Input: part model. Units: mm. Frame: model coordinates. A direction names the side the tool comes from. Coordinates: 2 decimals unless noted, no trailing zeros. Write each loop counter-clockwise with the first axis right and the second up, starting at its lowest first coordinate (ties: lowest second). Pieces come first, ordered by that corner, then holes.
Autodesk Inventor part; units mm, degrees
ref_plane "YZ Plane" through (0, 0, 0) normal (1, 0, 0) x (0, 1, 0)
ref_plane "XZ Plane" through (0, 0, 0) normal (0, 1, 0) x (-1, 0, 0)
ref_plane "XY Plane" through (0, 0, 0) normal (0, 0, 1) x (1, 0, 0)
sketch "Sketch2" plane through (0, 0, 0) normal (0, 1, 0) x (-1, 0, 0)
  line L0 (-2.5, 6) -> (2.5, 6)
  line L1 (2.5, 6) -> (2.5, -6)
  line L2 (2.5, -6) -> (-2.5, -6)
  line L3 (-2.5, -6) -> (-2.5, 6)
  line L4 (-2.5, 6) -> (2.5, -6) construction
  line L5 (2.5, 6) -> (-2.5, -6) construction
  line L6 (2.5, 0) -> (-2.5, 0)
  circle A0 centre (0, 3) radius 0.8
  circle A1 centre (0, -3) radius 0.8
  line L7 (-5.5, -9) -> (5.5, -9)
  line L8 (5.5, -9) -> (5.5, 9)
  line L9 (5.5, 9) -> (-5.5, 9)
  line L10 (-5.5, 9) -> (-5.5, -9)
  line L11 (-5.5, -9) -> (5.5, 9) construction
  line L12 (5.5, -9) -> (-5.5, 9) construction
  point P0 (0, 0)
  dimension "d2" = 5
  dimension "d3" = 12
  dimension "d4" = 1.6
  dimension "d5" = 2.5
  dimension "d6" = 3
  dimension "d7" = 11
  dimension "d8" = 18
extrude "Extrusion2" add sketch "Sketch2" along normal blind 2 contours L0 L1 L6 L3 | L6 L1 L2 L3
extrude "Extrusion3" add sketch "Sketch2" along normal blind 5 contours L10 L9 L8 L7
fillet "Fillet1" radius 2 8 edges at (-5.5, 0, 0) (0, 0, -9) (5.5, 0, 0) (0, 0, 9) (-5.5, 2.5, -9) (-5.5, 2.5, 9) (5.5, 2.5, 9) (5.5, 2.5, -9)
sketch "Sketch4" plane through (-5.5, 0, -9) normal (-1, 0, 0) x (0, 0, 1)
  line L0 (0, 0) -> (18, 0) construction
  line L1 (18, 0) -> (18, 5) construction
  line L2 (0, 0) -> (18, 0) construction
  line L3 (18, 0) -> (18, 2) construction
  line L4 (18, 2) -> (0, 2) construction
  line L5 (0, 2) -> (0, 0) construction
  line L6 (9, 0) -> (9, 7)
  line L7 (0, 5) -> (18, 5) construction
  circle A0 centre (6, 4.5) radius 1
  circle A1 centre (12, 4.5) radius 1
  dimension "d13" = 2
  dimension "d15" = 2
  dimension "d16" = 6
  dimension "d17" = 2.5
properties part number "Part1_3DPrint"
Item 1: Section query B-B, the plane x = 0.5. Return loops of the section in (y, z), then the cut area to 3 significant figures.
Item 2: Pin query (flat end, axial travel): pin 1 Ø4 at (x, z) = (0, 0.5) entering from +Y; pin 2 Ø1.3 at (x, z) = (0, -3) entering from +Y. Return the tip coordinate at first contact, or that it passes through.
Item 3: Section query A-A, the plane y = 4. Return loops of the section in (x, z).
Item 4: Material intervals for line 1 (X direction, y = 4.7, z = 4.5); line 2 (Z direction, x = 0, y = 1.25); line 3 (Z direction, x = 0.25, y = 4.15), sorted ascending.
Item 5: Section query D-D, the plane z = -0.75. Return loops of the section in (x, y).
Item 6: Pull-direction query (Z, two-part tool) for faces 1 (the face through (5.5, 3, 0)), 2 (the face through (0.17, 0.99, 3.78)), 3 (the face through (0.05, 0.6, 8.43)), 4 (the face through (0, 2, 0)); classes: released by +Z, released by -Z, zero draft, split by the parting line, or undercut.
Item 7: Access query for faces 5 (the face through (0, 3, -6)), 6 (the face through (0, 0, 0)). Directions: +Z, -Z, +X, -X, +Y, -Y. A direction counts if a zero-diameter tool reaches every point of the face in a straight line with its end or side. Return the directions, or none.
Item 8: Section query C-C, the plane z = 3. Return loops of the section in (x, y).
The answers:
1. outline: (0, -7) arc R2 ccw to (2, -9) - (5, -9) - (5, -6) - (2, -6) - (2, -3.62) - (0, -3.62) - close; (0, -2.38) - (2, -2.38) - (2, 2.38) - (0, 2.38) - close; (0, 3.62) - (2, 3.62) - (2, 6) - (5, 6) - (5, 9) - (2, 9) arc R2 ccw to (0, 7) - close
1. area: 47.3 mm2
2. pin 1: stops at y = 2
2. pin 2: passes through
3. outline: (-5.5, -7) arc R2 ccw to (-3.5, -9) - (3.5, -9) arc R2 ccw to (5.5, -7) - (5.5, 7) arc R2 ccw to (3.5, 9) - (-3.5, 9) arc R2 ccw to (-5.5, 7) - close; hole (-2.5, -6) - (2.5, -6) - (2.5, 6) - (-2.5, 6) - close
4. line 1: x = -5.5 to -2.5, 2.5 to 5.5
4. line 2: z = -8.85 to -3.8, -2.2 to 2.2, 3.8 to 8.85
4. line 3: z = -9 to -6, 6 to 9
5. outline: (-5.5, 2) arc R2 ccw to (-3.5, 0) - (3.5, 0) arc R2 ccw to (5.5, 2) - (5.5, 5) - (2.5, 5) - (2.5, 2) - (-2.5, 2) - (-2.5, 5) - (-5.5, 5) - close
6. face 1: zero draft
6. face 2: undercut
6. face 3: released by +Z
6. face 4: undercut
7. face 5: +Y
7. face 6: +Z, -Z, +X, -X, -Y
8. outline: (-5.5, 2) arc R2 ccw to (-3.5, 0) - (-0.8, 0) - (-0.8, 2) - (-2.5, 2) - (-2.5, 5) - (-5.5, 5) - close; (0.8, 0) - (3.5, 0) arc R2 ccw to (5.5, 2) - (5.5, 5) - (2.5, 5) - (2.5, 2) - (0.8, 2) - close
